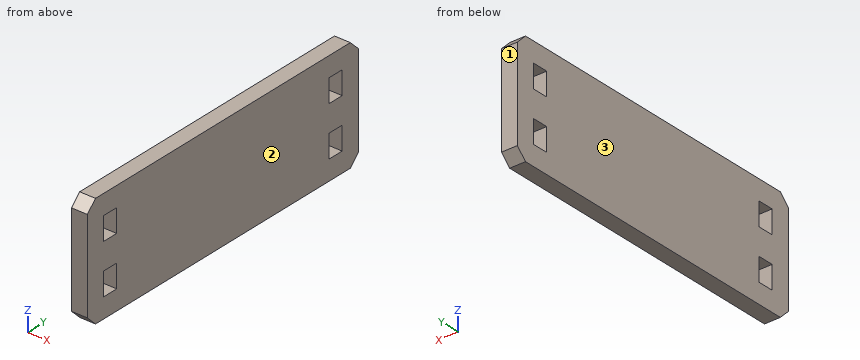
from build123d import *

# Parameters (mm, degrees)
SKETCH1_W           = 43.18
SKETCH1_H           = 126.492
SKETCH1_W_2         = 8.89
SKETCH1_H_2         = 6.096
BOSS_EXTRUDE1_DEPTH = 3.048
CHAMFER1_SIZE       = 3.81


with BuildPart() as part:
    # Sketch1 → Boss-Extrude1 (new body, symmetric)
    with BuildSketch(Plane(origin=(0, 0, 0), x_dir=(0, 0, -1), z_dir=(1, 0, 0))):
        with Locations((-111.027292876, 0)):
            Rectangle(SKETCH1_W, SKETCH1_H)
        with Locations((-101.502292876, 52.578)):
            Rectangle(SKETCH1_W_2, SKETCH1_H_2, mode=Mode.SUBTRACT)
        with Locations((-120.552292876, 52.578)):
            Rectangle(SKETCH1_W_2, SKETCH1_H_2, mode=Mode.SUBTRACT)
        with Locations((-101.502292876, -52.578)):
            Rectangle(SKETCH1_W_2, SKETCH1_H_2, mode=Mode.SUBTRACT)
        with Locations((-120.552292876, -52.578)):
            Rectangle(SKETCH1_W_2, SKETCH1_H_2, mode=Mode.SUBTRACT)
    extrude(amount=BOSS_EXTRUDE1_DEPTH, both=True)

    # Chamfer1
    chamfer1_edges = [part.edges().sort_by_distance(p)[0] for p in [
        (0, -63.246, 89.437292876),
        (0, -63.246, 132.617292876),
        (0, 63.246, 132.617292876),
        (0, 63.246, 89.437292876),
    ]]
    chamfer(chamfer1_edges, length=CHAMFER1_SIZE)


solid = part.part
Geometry: final body of the model. Coordinates: model frame, mm. Face numbers are marked on the shaded views. Round coordinates to 2 decimals unless told otherwise and drop trailing zeros. Loops run counter-clockwise (first coordinate to the right, second up) from the corner with the lowest first, then second, coordinate; pieces in that order, holes last. Notation, with made-up numbers: M -7.5,57.25 L 11.5,57.25 A30 ccw 11.5,83.25 Z; hole C 62,35 d7. An arc over 180 degrees is marked long. Put each result on its own line as item: value. Start each with the question number.
(1) Section query A-A (z = 119). Return loops of the section in (x, y).
(2) Material intervals for line 1 along Y through (x, z) = (2.5, 103.5); line 2 along Y through (x, z) = (2, 93), sorted ascending. Write a range as [from, to].
(3) Section query C-C (z = 130). Return loops of the section in (x, y), then the cut area to 3 significant figures.
(4) Section query B-B (x = 1.25). Return loops of the section in (y, z), then the cut area to 3 significant figures.
(5) Draft query along X for the marked faces 1, 2 and 3. Return one class per face: +X half, -X half, draft (parallel to the pull), parting line (faces both ways), or undercut.
Findings below:
1. outline: M -3.05,-63.25 L 3.05,-63.25 L 3.05,-55.63 L -3.05,-55.63 Z; M -3.05,-49.53 L 3.05,-49.53 L 3.05,49.53 L -3.05,49.53 Z; M -3.05,55.63 L 3.05,55.63 L 3.05,63.25 L -3.05,63.25 Z
2. line 1: y = [-63.25, -55.63], [-49.53, 49.53], [55.63, 63.25]
2. line 2: y = [-63, 63]
3. outline: M -3.05,-62.05 L 3.05,-62.05 L 3.05,62.05 L -3.05,62.05 Z
3. area: 757 mm2
4. outline: M -63.25,93.25 L -59.44,89.44 L 59.44,89.44 L 63.25,93.25 L 63.25,128.81 L 59.44,132.62 L -59.44,132.62 L -63.25,128.81 Z; hole M -55.63,97.06 L -49.53,97.06 L -49.53,105.95 L -55.63,105.95 Z; hole M -55.63,116.11 L -49.53,116.11 L -49.53,125 L -55.63,125 Z; hole M 49.53,97.06 L 55.63,97.06 L 55.63,105.95 L 49.53,105.95 Z; hole M 49.53,116.11 L 55.63,116.11 L 55.63,125 L 49.53,125 Z
4. area: 5,220 mm2
5. face 1: draft
5. face 2: +X half
5. face 3: -X half
